Could you check a few things on this model? Use its own coordinates, in mm. A direction names the side the tool comes from. Coordinates: 2 decimals unless noted, no trailing zeros. Write each loop counter-clockwise with the first axis right and the second up, starting at its lowest first coordinate (ties: lowest second). Pieces come first, ordered by that corner, then holes. Notation, with made-up numbers: (-5.75, 81.25) - (32.25, 81.25) arc R27 ccw to (32.25, 108.25) - close; hole circle Ø5 at (-16.75, -2.5). An arc over 180 degrees is marked (long way). Answer as a JSON object with one key per item and string values. Group by question number.
1) If we section it at D-D (z = -7.75): Write out the boundary of the cut face in (x, y), plus the area to 3 significant figures.
2) If we section it at B-B (x = 23): Write out the boundary of the cut face in (y, z), plus the area to 3 significant figures.
3) On a 3-axis mill with a long thin cutter (end or side, diameter ignored), from which of +Z, -Z, +X, -X, +Y, -Y can I reach the whole of each face in a straight line? I mean faces 1 (the flat face through (0, 27.813, 7)), 2 (the flat face through (0, -5, 14.478)), 3 (the flat face through (0, -6, -2.377)). Say none if no direction works.
4) If we section it at A-A (z = 1.5): Write out the boundary of the cut face in (x, y).
5) If we section it at C-C (y = 11.5): Write out the boundary of the cut face in (x, z).
6) Please list where these lines run through material, in increasing order: line 1 along Z through (x, y) = (-25, 2); line 2 along Y through (x, z) = (-19, 9.5); line 3 along Y through (x, z) = (-19, 4).
7) Will these pins go through, and if not, where does the flat tip stop? pin 1 Ø12 at (x, z) = (-5, -4) entering from -Y; pin 2 Ø6 at (x, y) = (-12.5, -17) entering from -Z; pin 3 Ø16 at (x, z) = (-12.5, 9) entering from +Y; pin 4 Ø11.5 at (x, z) = (4.5, 9) entering from -Y.
```python
from build123d import *

# Parameters (mm, degrees)
F0_W     = 55.626
F0_H     = 55.626
F1_DEPTH = 14.478
F2_W     = 55.626
F2_H     = 14.478
F3_DEPTH = 10.16
F5_DEPTH = 55.626


with BuildPart() as f1:
    # F0 (on Top) → F1 (new body)
    with BuildSketch(Plane.XY):
        Rectangle(F0_W, F0_H)
    extrude(amount=F1_DEPTH)

    # F2 (on face) → F3 (join)
    with BuildSketch(Plane.XZ.offset(27.813)):
        with Locations((0, 7.239)):
            Rectangle(F2_W, F2_H)
    extrude(amount=F3_DEPTH)

    # F4 (on face) → F5 (join)
    with BuildSketch(Plane(origin=(-27.813, 0, 0), x_dir=(0, -1, 0), z_dir=(-1, 0, 0))):
        Polygon((37.973, 0), (-27.813, 0), (-32.288288, -11.885361), (-29.911216, -12.780418), (-25.993962, -2.377072), (39.792038, -2.377072), (40.687095, 0), (45.427891, 12.59049), (43.050819, 13.485548), align=None)
    extrude(amount=-F5_DEPTH)


solid = f1.part
```
Here are the results:
{
 "1": {"outline": "(-27.81, 28.02) - (27.81, 28.02) - (27.81, 30.73) - (-27.81, 30.73) - close", "area": "151 mm²"},
 "2": {"outline": "(-45.43, 12.59) - (-40.69, 0) - (-39.79, -2.38) - (25.99, -2.38) - (29.91, -12.78) - (32.29, -11.89) - (27.81, 0) - (27.81, 14.48) - (-37.97, 14.48) - (-37.97, 0) - (-43.05, 13.49) - close", "area": "1,180 mm²"},
 "3": {"face 1": "+Z, +X, -X, +Y", "face 2": "+Z, +X, -X, +Y, -Y", "face 3": "-Z, +X, -X, -Y"},
 "4": {"outline": "(-27.81, -41.25) - (27.81, -41.25) - (27.81, -38.54) - (-27.81, -38.54) - close; (-27.81, -37.97) - (27.81, -37.97) - (27.81, 27.81) - (-27.81, 27.81) - close"},
 "5": {"outline": "(-27.81, -2.38) - (27.81, -2.38) - (27.81, 14.48) - (-27.81, 14.48) - close"},
 "6": {"line 1": "z = -2.38 to 14.48", "line 2": "y = -44.26 to -41.55, -37.97 to 27.81", "line 3": "y = -42.19 to -39.48, -37.97 to 27.81"},
 "7": {"pin 1": "stops at y = -41.44", "pin 2": "stops at z = -2.38", "pin 3": "stops at y = 27.81", "pin 4": "stops at y = -45.43"}
}
